```python
from build123d import *

# Parameters (mm, degrees)
SKETCH2_R           = 2.4
BOSS_EXTRUDE1_DEPTH = 8
SKETCH3_R           = 3.1
CUT_EXTRUDE1_DEPTH  = 1


with BuildPart() as part:
    # Sketch2 → Boss-Extrude1 (new body)
    with BuildSketch(Plane.XY):
        with BuildLine():
            Line((3.9, 3.3), (-4.797530266, 3.3))
            ThreePointArc((-4.797530266, 3.3), (-8.097530266, 0), (-4.797530266, -3.3))
            Line((-4.797530266, -3.3), (3.9, -3.3))
            ThreePointArc((3.9, -3.3), (7.2, 0), (3.9, 3.3))
        make_face()
        with Locations((3.9, 0)):
            Circle(SKETCH2_R, mode=Mode.SUBTRACT)
        with BuildLine():
            Line((-6.975235481, 0.84), (-6.037530266, 0.84))
            ThreePointArc((-6.037530266, 0.84), (-5.754687554, 0.957157288), (-5.637530266, 1.24))
            Line((-5.637530266, 1.24), (-5.637530266, 2.177705214))
            ThreePointArc((-5.637530266, 2.177705214), (-5.618824151, 2.235940121), (-5.56970418, 2.27238805))
            ThreePointArc((-5.56970418, 2.27238805), (-4.797530266, 2.4), (-4.025356353, 2.27238805))
            ThreePointArc((-4.025356353, 2.27238805), (-3.976236382, 2.235940121), (-3.957530266, 2.177705214))
            Line((-3.957530266, 2.177705214), (-3.957530266, 1.24))
            ThreePointArc((-3.957530266, 1.24), (-3.840372979, 0.957157288), (-3.557530266, 0.84))
            Line((-3.557530266, 0.84), (-2.619825052, 0.84))
            Line((-2.619825052, 0.84), (-2.549330987, 0.84))
            Line((-2.549330987, 0.84), (-1.35081169, 0.84))
            ThreePointArc((-1.35081169, 0.84), (-1.557752494, 1.445797742), (-1.870126582, 2.004580194))
            ThreePointArc((-1.870126582, 2.004580194), (-1.919033599, 2.358251088), (-1.665957447, 2.610099174))
            ThreePointArc((-1.665957447, 2.610099174), (-0.8, 2.75), (0.065957447, 2.610099174))
            ThreePointArc((0.065957447, 2.610099174), (0.319033599, 2.358251088), (0.270126582, 2.004580194))
            ThreePointArc((0.270126582, 2.004580194), (-0.35, 0), (0.270126582, -2.004580194))
            ThreePointArc((0.270126582, -2.004580194), (0.319033599, -2.358251088), (0.065957447, -2.610099174))
            ThreePointArc((0.065957447, -2.610099174), (-0.8, -2.75), (-1.665957447, -2.610099174))
            ThreePointArc((-1.665957447, -2.610099174), (-1.919033599, -2.358251088), (-1.870126582, -2.004580194))
            ThreePointArc((-1.870126582, -2.004580194), (-1.557752494, -1.445797742), (-1.35081169, -0.84))
            Line((-1.35081169, -0.84), (-2.549330987, -0.84))
            Line((-2.549330987, -0.84), (-2.619825052, -0.84))
            Line((-2.619825052, -0.84), (-3.557530266, -0.84))
            ThreePointArc((-3.557530266, -0.84), (-3.840372979, -0.957157288), (-3.957530266, -1.24))
            Line((-3.957530266, -1.24), (-3.957530266, -2.177705214))
            ThreePointArc((-3.957530266, -2.177705214), (-3.976236382, -2.235940121), (-4.025356353, -2.27238805))
            ThreePointArc((-4.025356353, -2.27238805), (-4.797530266, -2.4), (-5.56970418, -2.27238805))
            ThreePointArc((-5.56970418, -2.27238805), (-5.618824151, -2.235940121), (-5.637530266, -2.177705214))
            Line((-5.637530266, -2.177705214), (-5.637530266, -1.24))
            ThreePointArc((-5.637530266, -1.24), (-5.754687554, -0.957157288), (-6.037530266, -0.84))
            Line((-6.037530266, -0.84), (-6.975235481, -0.84))
            ThreePointArc((-6.975235481, -0.84), (-7.033470387, -0.821293884), (-7.069918316, -0.772173913))
            ThreePointArc((-7.069918316, -0.772173913), (-7.197530266, 0), (-7.069918316, 0.772173913))
            ThreePointArc((-7.069918316, 0.772173913), (-7.033470387, 0.821293884), (-6.975235481, 0.84))
        make_face(mode=Mode.SUBTRACT)
    extrude(amount=BOSS_EXTRUDE1_DEPTH)

    # Sketch3 → Cut-Extrude1 (cut)
    with BuildSketch(Plane.XY.offset(8)):
        with Locations((3.9, 0)):
            Circle(SKETCH3_R)
    cut_extrude1 = extrude(amount=-CUT_EXTRUDE1_DEPTH, mode=Mode.SUBTRACT)

    # Mirror1: Cut-Extrude1 across plane
    add(cut_extrude1.mirror(Plane.XY.offset(4)), mode=Mode.SUBTRACT)


solid = part.part
```
The listing builds one solid part. Answer for the finished solid, in the listing's coordinates (mm). A direction names the side the tool comes from. Give positions to 0.01 mm unless a question says otherwise; leave off trailing zeros. Loops run counter-clockwise (first coordinate to the right, second up) from the corner with the lowest first, then second, coordinate; pieces in that order, holes last. Notation, with made-up numbers: M -12,89 L 25,89 A19 ccw 25,107 Z; hole C -4,51.25 d1. An arc over 180 degrees is marked long. One line per item, written item: value.
1. For a pull along X with two mould halves and no side action, classify faces 4 (the face through (-1.56, -1.45, 3.94)), 5 (the face through (-2.3, 1.5, 0)), 6 (the face through (7.2, -0.1, 3.9)) as pulls with the +X half, pulls with the -X half, needs draft (parallel to the pull), parting line crosses it, or undercut.
Found:
face 4: undercut
face 5: needs draft
face 6: pulls with the +X half
2. Section A-A on x = -2.75 is taken. Determine the outline of the cut face in (y, z).
Found:
outline: M -3.3,0 L -0.84,0 L -0.84,8 L -3.3,8 Z; M 0.84,0 L 3.3,0 L 3.3,8 L 0.84,8 Z
3. Find the intervals of material crossed by probe 1 along X at (y, z) = (0, 4.5); probe 2 along Y at (x, z) = (0, 7.5); probe 3 along X at (y, z) = (-2, 6), in increasing order.
Found:
probe 1: -8.1 to -7.2, -0.35 to 1.5, 6.3 to 7.2
probe 2: -3.3 to -2.63, -1.54 to 1.54, 2.63 to 3.3
probe 3: -7.42 to -5.64, -3.96 to -1.87, 0.27 to 2.57, 5.23 to 6.52
4. Section D-D on x = -4.5 is taken. Determine the outline of the cut face in (y, z).
Found:
outline: M -3.3,0 L -2.38,0 L -2.38,8 L -3.3,8 Z; M 2.38,0 L 3.3,0 L 3.3,8 L 2.38,8 Z
5. For faces 1 (the face through (5.33, -2.75, 7.51)), 2 (the face through (-2.3, 1.5, 8)), 3 (the face through (-1.554, 1.438, 3.944)), determine the directions among +Z, -Z, +X, -X, +Y, -Y from which every point of the face is accessible in a straight line to the end or side of a thin tool.
Found:
face 1: +Z
face 2: +Z, +X, -X, +Y, -Y
face 3: +Z, -Z
6. Section C-C on z = 6.5 is taken. State how many separate pieces and enclosed holes the cut face has, plus the area to 3 significant figures.
Found:
separate pieces: 1
enclosed holes: 2
area: 50.3 mm^2
7. Each of these flat-tipped pins is pushed along its axis until it touches: P1, Ø0.8, axis at x = -6.5, z = 2.5, coming from the +Y side; P2, Ø0.5, axis at y = -2, z = 3.5, coming from the -X side; P3, Ø1.9, axis at x = 4, y = -0.5, coming from the +Z side. Where does it stop, or does it pass through?
Found:
P1: y = 3.03
P2: x = -7.6
P3: through
8. Section B-B on y = 0 is taken. Determine the outline of the cut face in (x, z).
Found:
outline: M -8.1,0 L -7.2,0 L -7.2,8 L -8.1,8 Z; M -0.35,0 L 0.8,0 L 0.8,1 L 1.5,1 L 1.5,7 L 0.8,7 L 0.8,8 L -0.35,8 Z; M 6.3,1 L 7,1 L 7,0 L 7.2,0 L 7.2,8 L 7,8 L 7,7 L 6.3,7 Z
